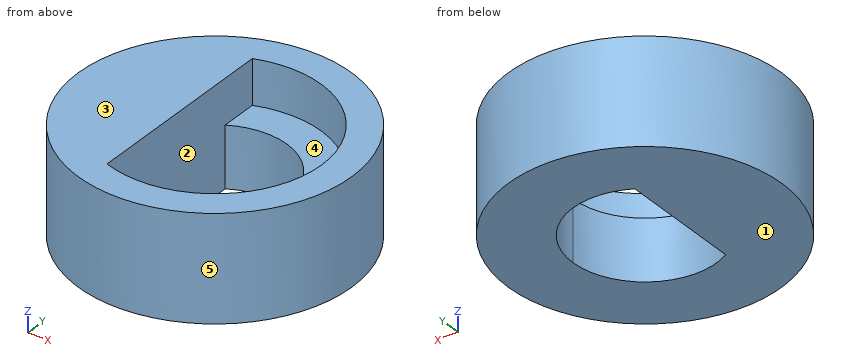
```python
from build123d import *

# Parameters (mm, degrees)
F1_DEPTH = 3
F0_R     = 6.75
F2_DEPTH = 5.2


with BuildPart() as f1:
    # F0 (on Top) → F1 (new body)
    with BuildSketch(Plane.XY):
        with BuildLine():
            ThreePointArc((-1.745, 3.0972568508), (1.7936763922, 3.0693240298), (3.555, 0))
            ThreePointArc((3.555, 0), (1.7936763922, -3.0693240298), (-1.745, -3.0972568508))
            Line((-1.745, -3.0972568508), (-1.745, -4.9515123952))
            ThreePointArc((-1.745, -4.9515123952), (3.0332532041, -4.2850758453), (5.25, 0))
            ThreePointArc((5.25, 0), (3.0332532041, 4.2850758453), (-1.745, 4.9515123952))
            Line((-1.745, 4.9515123952), (-1.745, 3.0972568508))
        make_face()
    extrude(amount=F1_DEPTH)

    # F0 (on Top) → F2 (join)
    with BuildSketch(Plane.XY):
        Circle(F0_R)
        with BuildLine():
            ThreePointArc((-1.745, -4.9515123952), (-5.25, 0), (-1.745, 4.9515123952))
            ThreePointArc((-1.745, 4.9515123952), (3.0332532041, 4.2850758453), (5.25, 0))
            ThreePointArc((5.25, 0), (3.0332532041, -4.2850758453), (-1.745, -4.9515123952))
        make_face(mode=Mode.SUBTRACT)
        with BuildLine():
            ThreePointArc((-1.745, -3.0972568508), (-3.555, 0), (-1.745, 3.0972568508))
            Line((-1.745, 3.0972568508), (-1.745, 4.9515123952))
            ThreePointArc((-1.745, 4.9515123952), (-5.25, 0), (-1.745, -4.9515123952))
            Line((-1.745, -4.9515123952), (-1.745, -3.0972568508))
        make_face()
        with BuildLine():
            Line((-1.745, 0), (-1.745, 3.0972568508))
            ThreePointArc((-1.745, 3.0972568508), (-3.555, 0), (-1.745, -3.0972568508))
            Line((-1.745, -3.0972568508), (-1.745, 0))
        make_face()
    extrude(amount=F2_DEPTH)


solid = f1.part
```
Source: CAD feature listing. Evaluate the final solid. Frame: model axes, mm. Face numbers are marked on the shaded views. A direction names the side the tool comes from. Round coordinates to 2 decimals unless told otherwise and drop trailing zeros. Loops run counter-clockwise (first coordinate to the right, second up) from the corner with the lowest first, then second, coordinate; pieces in that order, holes last. Notation, with made-up numbers: M -23.75,79.25 L -18.75,79.25 A15 ccw -18.75,99.25 Z; hole C 6.25,35 d2. An arc over 180 degrees is marked long. Use a Markdown table: item, result. Add a question column.
1. Cut plane A-A, the plane y = 2. Output: boundary loops of the cut face in (x, z) (3 decimals).
2. Set-up query: the marked faces 1 and 2. Return all of +Z, -Z, +X, -X, +Y, -Y with unobstructed straight access to the full face (end or side cutting, diameter ignored); none if empty.
3. Cut plane C-C, the plane z = 3.6. Output: boundary loops of the cut face in (x, y) (3 decimals), and give its area (3 significant figures).
4. Pull-direction query (Y, two-part tool) for the marked faces 3, 4 and 5; classes: +Y half, -Y half, draft (parallel to the pull), parting line (faces both ways), or undercut.
5. Contact query for flat-ended pins moving along their axis: pin 1 (1 mm diameter, centred on x = 4.5, z = 1, fed in from -Y); pin 2 (1 mm diameter, centred on y = -3.5, z = 4, fed in from +X); pin 3 (1 mm diameter, centred on x = -4, z = 3.5, fed in from +Y). Output: stop coordinate, or through.
6. Cut plane D-D, the plane x = 0. Output: boundary loops of the cut face in (y, z) (3 decimals), and give its area (3 significant figures).
7. Cut plane B-B, the plane x = 1.75. Output: boundary loops of the cut face in (y, z).
8. Ray query, line 1 along Z through (x, y) = (4.25, -2); line 2 along X through (y, z) = (-3.25, 4.6) (3 decimals); line 3 along X through (y, z) = (-1.75, 1.15) (3 decimals). Return the intervals inside material, ascending. Write a range as [from, to].
Solution:
| question | item | result |
|---|---|---|
| 1 | outline | M -6.447,0 L -1.745,0 L -1.745,5.2 L -6.447,5.2 Z; M 2.939,0 L 6.447,0 L 6.447,5.2 L 4.854,5.2 L 4.854,3 L 2.939,3 Z |
| 2 | face 1 | -Z, +X, -X, +Y, -Y |
| 2 | face 2 | +Z |
| 3 | outline | C 0,0 d13.5; hole M -1.745,-4.952 A5.25 ccw long -1.745,4.952 Z |
| 3 | area | 81.9 mm2 |
| 4 | face 3 | draft |
| 4 | face 4 | undercut |
| 4 | face 5 | parting line |
| 5 | pin 1 | stops at y = -5.44 |
| 5 | pin 2 | stops at x = 6.05 |
| 5 | pin 3 | stops at y = 5.77 |
| 6 | outline | M -6.75,0 L -3.555,0 L -3.555,3 L -5.25,3 L -5.25,5.2 L -6.75,5.2 Z; M 3.555,0 L 6.75,0 L 6.75,5.2 L 5.25,5.2 L 5.25,3 L 3.555,3 Z |
| 6 | area | 25.8 mm2 |
| 7 | outline | M -6.52,0 L -3.09,0 L -3.09,3 L -4.95,3 L -4.95,5.2 L -6.52,5.2 Z; M 3.09,0 L 6.52,0 L 6.52,5.2 L 4.95,5.2 L 4.95,3 L 3.09,3 Z |
| 8 | line 1 | z = [0, 3] |
| 8 | line 2 | x = [-5.916, -1.745], [4.123, 5.916] |
| 8 | line 3 | x = [-6.519, -1.745], [3.094, 6.519] |
